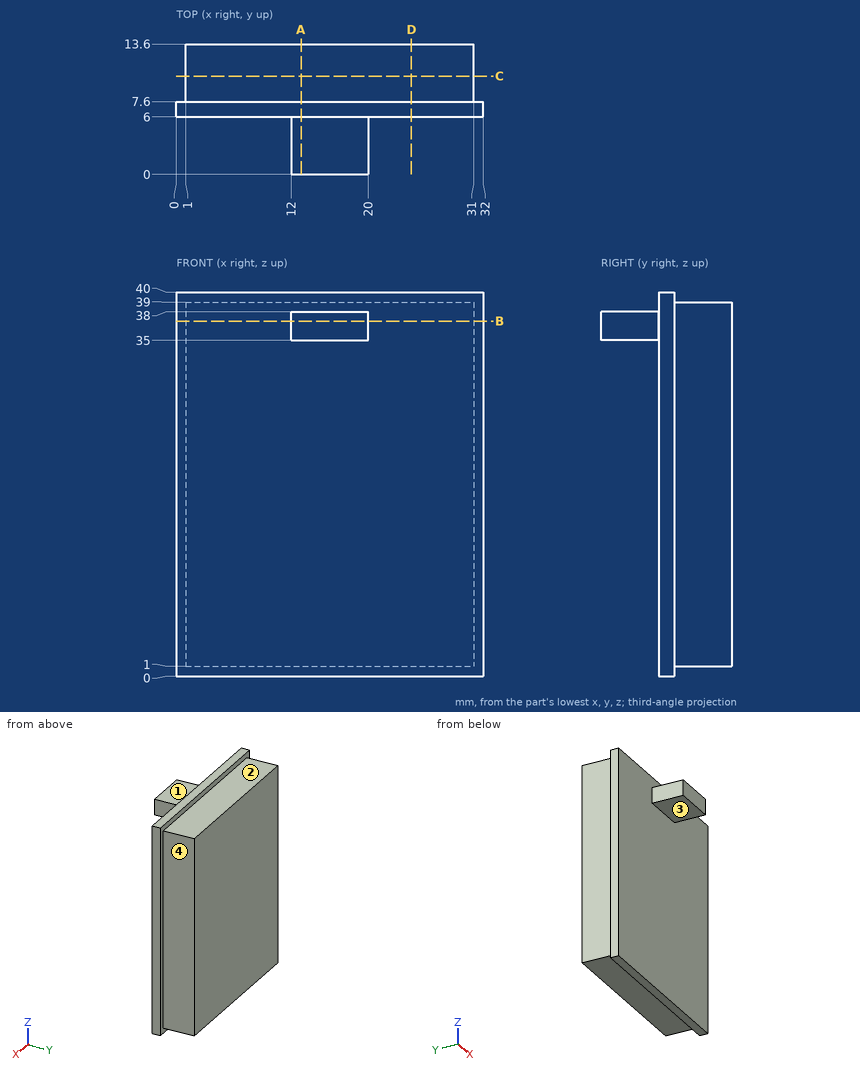
Geometry check sheet. Reference: drawing and pictorial views, mm from the part's lowest x, y, z. A direction names the side the tool comes from. Give positions to 0.01 mm unless a question says otherwise; leave off trailing zeros. Write each loop counter-clockwise with the first axis right and the second up, starting at its lowest first coordinate (ties: lowest second). Pieces come first, ordered by that corner, then holes. Notation, with made-up numbers: (2.25, 65) -> (31.25, 65) arc R29 ccw to (31.25, 91) -> close; hole circle Ø1 at (1, 46). An arc over 180 degrees is marked (long way). One line per item, written item: value. Start each with the question number.
Item 1: Material ranges on probe 1 along Z at (x, y) = (15.5, 2.5); probe 2 along Z at (x, y) = (4.5, 12.5); probe 3 along Y at (x, z) = (9, 9.5), recorded low to high. Write a range as from..to.
Item 2: Section check B-B on z = 37. Record the cut outline in (x, y), then the cut area to 3 significant figures.
Item 3: Tool access check on the marked faces 1, 2, 3 and 4. Record the directions out of +Z, -Z, +X, -X, +Y, -Y that give a thin tool (end or side, any length) a straight path to the whole face; none if there is none.
Item 4: Gauge pin test, flat ends, axial feed: pin 1 (5 mm diameter, centred on x = 16.5, y = 1.5, fed in from -Z); pin 2 (3 mm diameter, centred on x = 19.5, y = 10.5, fed in from +Z); pin 3 (3 mm diameter, centred on y = 10.5, z = 24, fed in from -X). Record the tip position at first contact, or that the pin passes through.
Item 5: Section check C-C on y = 10.25. Record the cut outline in (x, z).
Item 6: Section check A-A on x = 13. Record the cut outline in (y, z), then the cut area to 3 significant figures.
Item 7: Section check D-D on x = 24.5. Record the cut outline in (y, z), then the cut area to 3 significant figures.
Results list:
1. probe 1: 35..38
1. probe 2: 1..39
1. probe 3: 6..13.6
2. outline: (0, 6) -> (12, 6) -> (12, 0) -> (20, 0) -> (20, 6) -> (32, 6) -> (32, 7.6) -> (31, 7.6) -> (31, 13.6) -> (1, 13.6) -> (1, 7.6) -> (0, 7.6) -> close
2. area: 279 mm²
3. face 1: +Z, +X, -X, -Y
3. face 2: +Z, +X, -X, +Y
3. face 3: -Z, +X, -X, -Y
3. face 4: +Z, -Z, +X, +Y
4. pin 1: z = 35
4. pin 2: z = 39
4. pin 3: x = 1
5. outline: (1, 1) -> (31, 1) -> (31, 39) -> (1, 39) -> close
6. outline: (0, 35) -> (6, 35) -> (6, 0) -> (7.6, 0) -> (7.6, 1) -> (13.6, 1) -> (13.6, 39) -> (7.6, 39) -> (7.6, 40) -> (6, 40) -> (6, 38) -> (0, 38) -> close
6. area: 310 mm²
7. outline: (6, 0) -> (7.6, 0) -> (7.6, 1) -> (13.6, 1) -> (13.6, 39) -> (7.6, 39) -> (7.6, 40) -> (6, 40) -> close
7. area: 292 mm²
